Input: part model. Units: mm. Frame: model coordinates. A direction names the side the tool comes from. Coordinates: 2 decimals unless noted, no trailing zeros. Loops run counter-clockwise (first coordinate to the right, second up) from the corner with the lowest first, then second, coordinate; pieces in that order, holes last. Notation, with made-up numbers: (48, -10.5) -> (107, -10.5) arc R22 ccw to (107, 26.5) -> close; hole circle Ø7 at (-32.75, 14.5). An arc over 180 degrees is marked (long way). Answer as a JSON object with one key per item and string values.
from build123d import *

# Parameters (mm, degrees)
BOSS_EXTRUDE1_DEPTH  = 1
SKETCH2_W            = 16
SKETCH2_H            = 10
BOSS_EXTRUDE2_DEPTH  = 10
SKETCH3_W            = 4.889113018
SKETCH3_H            = 5.37802432
CUT_EXTRUDE1_DEPTH   = 10
SKETCH4_W            = 45
SKETCH4_H            = 2.4
SKETCH4_W_2          = 30
BOSS_EXTRUDE3_DEPTH  = 4
SKETCH5_W            = 35
SKETCH5_H            = 10
BOSS_EXTRUDE4_DEPTH  = 7
SKETCH6_W            = 35
SKETCH6_H            = 1.5
CUT_EXTRUDE2_DEPTH   = 4
FILLET1_R            = 1
SKETCH7_R            = 1.5
CUT_EXTRUDE3_DEPTH   = 4
SKETCH8_W            = 0.75
SKETCH8_H            = 0.75
BOSS_EXTRUDE5_DEPTH  = 6
LPATTERN1_COUNT      = 10
LPATTERN1_PITCH      = 3
SKETCH9_W            = 0.75
SKETCH9_H            = 0.75
BOSS_EXTRUDE6_DEPTH  = 6
LPATTERN2_COUNT      = 15
LPATTERN2_PITCH      = 3
SKETCH10_R           = 2.5
BOSS_EXTRUDE7_DEPTH  = 6
SKETCH11_W           = 4.8
SKETCH11_H           = 9
BOSS_EXTRUDE8_DEPTH  = 4
SKETCH12_W           = 0.75
SKETCH12_H           = 0.75
BOSS_EXTRUDE9_DEPTH  = 6
LPATTERN3_COUNT      = 3
LPATTERN3_PITCH      = 3
LPATTERN3_COUNT_DIR2 = 2
LPATTERN3_PITCH_DIR2 = 3
SKETCH13_W           = 14.120912951
SKETCH13_H           = 4.362558473
BOSS_EXTRUDE10_DEPTH = 4
FILLET2_R            = 1


with BuildPart() as part:
    # Sketch1 → Boss-Extrude1 (new body)
    with BuildSketch(Plane.XY):
        Polygon((22.754016647, 124.270947632), (19.754016647, 127.270947632), (-45.245983353, 127.270947632), (-45.245983353, 74.270947632), (19.754016647, 74.270947632), (19.754016647, 90.113910289), (22.754016647, 92.500164177), align=None)
    extrude(amount=-BOSS_EXTRUDE1_DEPTH)

    # Sketch2 → Boss-Extrude2 (add)
    with BuildSketch(Plane(origin=(0, 0, -1), x_dir=(-1, 0, 0), z_dir=(0, 0, -1))):
        with Locations((46.316496684, 91.208096568)):
            Rectangle(SKETCH2_W, SKETCH2_H)
    extrude(amount=BOSS_EXTRUDE2_DEPTH)

    # Sketch3 → Cut-Extrude1 (cut)
    with BuildSketch(Plane.ZY.offset(54.316496684)):
        with Locations((-6.06540843, 91.2419286)):
            Rectangle(SKETCH3_W, SKETCH3_H)
    extrude(amount=-CUT_EXTRUDE1_DEPTH, mode=Mode.SUBTRACT)

    # Sketch4 → Boss-Extrude3 (add)
    with BuildSketch(Plane(origin=(0, 0, -1), x_dir=(-1, 0, 0), z_dir=(0, 0, -1))):
        with Locations((5.745983353, 77.470947632)):
            Rectangle(SKETCH4_W, SKETCH4_H)
        with Locations((-0.254016647, 124.070947632)):
            Rectangle(SKETCH4_W_2, SKETCH4_H)
    extrude(amount=BOSS_EXTRUDE3_DEPTH)

    # Sketch5 → Boss-Extrude4 (add)
    with BuildSketch(Plane(origin=(0, 0, -1), x_dir=(-1, 0, 0), z_dir=(0, 0, -1))):
        with Locations((3.745983353, 113.370947632)):
            Rectangle(SKETCH5_W, SKETCH5_H)
    extrude(amount=BOSS_EXTRUDE4_DEPTH)

    # Sketch6 → Cut-Extrude2 (cut)
    with BuildSketch(Plane(origin=(0, 0, -8), x_dir=(-1, 0, 0), z_dir=(0, 0, -1))):
        with Locations((3.745983353, 117.620947632)):
            Rectangle(SKETCH6_W, SKETCH6_H)
        with Locations((3.745983353, 109.120947632)):
            Rectangle(SKETCH6_W, SKETCH6_H)
    extrude(amount=-CUT_EXTRUDE2_DEPTH, mode=Mode.SUBTRACT)

    # Fillet1
    fillet1_edges = [part.edges().sort_by_distance(p)[0] for p in [
        (13.754016647, 109.870947632, -6),
        (-21.245983353, 109.870947632, -6),
        (13.754016647, 116.870947632, -6),
        (-21.245983353, 116.870947632, -6),
    ]]
    fillet(fillet1_edges, radius=FILLET1_R)

    # Sketch7 → Cut-Extrude3 (cut)
    with BuildSketch(Plane(origin=(0, 0, -1), x_dir=(-1, 0, 0), z_dir=(0, 0, -1))):
        with Locations((-17.700101194, 119.270947632)):
            Circle(SKETCH7_R)
        with Locations((-17.700101194, 91.270947632)):
            Circle(SKETCH7_R)
        with Locations((33.799898806, 125.270947632)):
            Circle(SKETCH7_R)
        with Locations((33.799898806, 77.270947632)):
            Circle(SKETCH7_R)
    extrude(amount=-CUT_EXTRUDE3_DEPTH, mode=Mode.SUBTRACT)

    # Sketch8 → Boss-Extrude5 (add)
    with BuildSketch(Plane(origin=(0, 0, -5), x_dir=(-1, 0, 0), z_dir=(0, 0, -1))):
        with Locations((-13.879016647, 124.070947632)):
            Rectangle(SKETCH8_W, SKETCH8_H)
    boss_extrude5 = extrude(amount=BOSS_EXTRUDE5_DEPTH)

    # LPattern1: Boss-Extrude5 ×10
    with Locations(*[(-i * LPATTERN1_PITCH, 0, 0) for i in range(1, LPATTERN1_COUNT)]):
        add(boss_extrude5)

    # Sketch9 → Boss-Extrude6 (add)
    with BuildSketch(Plane(origin=(0, 0, -5), x_dir=(-1, 0, 0), z_dir=(0, 0, -1))):
        with Locations((-15.402792453, 77.470947632)):
            Rectangle(SKETCH9_W, SKETCH9_H)
    boss_extrude6 = extrude(amount=BOSS_EXTRUDE6_DEPTH)

    # LPattern2: Boss-Extrude6 ×15
    with Locations(*[(-i * LPATTERN2_PITCH, 0, 0) for i in range(1, LPATTERN2_COUNT)]):
        add(boss_extrude6)

    # Sketch10 → Boss-Extrude7 (add)
    with BuildSketch(Plane(origin=(0, 0, -1), x_dir=(-1, 0, 0), z_dir=(0, 0, -1))):
        with Locations((26.546732083, 118.214976991)):
            Circle(SKETCH10_R)
        with Locations((31.940661119, 118.214976991)):
            Circle(SKETCH10_R)
    extrude(amount=BOSS_EXTRUDE7_DEPTH)

    # Sketch11 → Boss-Extrude8 (add)
    with BuildSketch(Plane(origin=(0, 0, -1), x_dir=(-1, 0, 0), z_dir=(0, 0, -1))):
        with Locations((-19.349242758, 100.613910289)):
            Rectangle(SKETCH11_W, SKETCH11_H)
    extrude(amount=BOSS_EXTRUDE8_DEPTH)

    # Sketch12 → Boss-Extrude9 (add)
    with BuildSketch(Plane(origin=(0, 0, -5), x_dir=(-1, 0, 0), z_dir=(0, 0, -1))):
        with Locations((-20.624242758, 97.488910289)):
            Rectangle(SKETCH12_W, SKETCH12_H)
    boss_extrude9 = extrude(amount=BOSS_EXTRUDE9_DEPTH)

    # LPattern3: Boss-Extrude9 3 × 2
    with Locations(*[(-j * LPATTERN3_PITCH_DIR2, i * LPATTERN3_PITCH, 0) for i in range(LPATTERN3_COUNT) for j in range(LPATTERN3_COUNT_DIR2) if (i, j) != (0, 0)]):
        add(boss_extrude9)

    # Sketch13 → Boss-Extrude10 (add)
    with BuildSketch(Plane(origin=(0, 0, -1), x_dir=(-1, 0, 0), z_dir=(0, 0, -1))):
        with Locations((23.447660741, 101.747194556)):
            Rectangle(SKETCH13_W, SKETCH13_H)
    extrude(amount=BOSS_EXTRUDE10_DEPTH)

    # Fillet2
    fillet2_edges = [part.edges().sort_by_distance(p)[0] for p in [
        (-16.387204265, 103.928473792, -3),
        (-16.387204265, 99.565915319, -3),
        (-30.508117216, 99.565915319, -3),
        (-30.508117216, 103.928473792, -3),
    ]]
    fillet(fillet2_edges, radius=FILLET2_R)


solid = part.part
1. Section query C-C (y = 95). Return loops of the section in (x, z).
Reply:
{"outline": "(-54.32, -11) -> (-38.32, -11) -> (-38.32, -1) -> (22.75, -1) -> (22.75, 0) -> (-45.25, 0) -> (-45.25, -1) -> (-54.32, -1) -> close"}
2. Section query A-A (x = -40). Return loops of the section in (y, z), plus the area to 3 significant figures.
Reply:
{"outline": "(74.27, -1) -> (86.21, -1) -> (86.21, -11) -> (96.21, -11) -> (96.21, -1) -> (127.27, -1) -> (127.27, 0) -> (74.27, 0) -> close", "area": "153 mm2"}
3. Line query: line 1 along Y through (x, z) = (2.5, -2); line 2 along X through (y, z) = (117, -3); line 3 along X through (y, z) = (100.5, -6.5). Output: solid intervals per line, ascending.
Reply:
{"line 1": "y = 76.27 to 78.67, 108.37 to 118.37, 122.87 to 125.27", "line 2": "x = -34.13 to -29.76, -28.73 to -24.36, -21.25 to 13.75", "line 3": "x = 17.25 to 18, 20.25 to 21"}
4. Section query D-D (y = 122). Return loops of the section in (x, z).
Reply:
{"outline": "(-45.25, -1) -> (22.75, -1) -> (22.75, 0) -> (-45.25, 0) -> close"}
5. Section query B-B (z = -9.5). Count the separate pieces of the cut face and the enclosed holes in it, plus the area to 3 significant figures.
Reply:
{"separate pieces": "32", "enclosed holes": "0", "area": "177 mm2"}
6. Access query for faces 4 (the face through (16.949, 101, -3)), 5 (the face through (-49, 91, -8.51)), 6 (the face through (-26.005, 115.774, -3.958)). Directions: +Z, -Z, +X, -X, +Y, -Y. A direction counts if a zero-diameter tool reaches every point of the face in a straight line with its end or side. Return the directions, or none.
Reply:
{"face 4": "-Z, +Y, -Y", "face 5": "-X", "face 6": "-Z"}
7. Pin query (flat end, axial travel): P1, Ø0.8, axis at x = 5, z = -8.5, coming from the -Y side; P2, Ø10, axis at x = 12.5, y = 85, coming from the +Z side; P3, Ø0.6, axis at x = -14.5, z = -7.5, coming from the -Y side; P4, Ø6, axis at x = -34, y = 89.5, coming from the -Z side. Return the tip coordinate at first contact, or that it passes through.
Reply:
{"P1": "stops at y = 123.7", "P2": "stops at z = 0", "P3": "stops at y = 77.1", "P4": "stops at z = -1"}
8. Mould query, pull axis Y, two halves, no side actions, for faces 1 (the face through (-30.508, 102, -3)), 2 (the face through (21.23, 91.29, -0.49)), 3 (the face through (-5, 78.671, -3)). Classes: pulls with the +Y half, pulls with the -Y half, needs draft (parallel to the pull), parting line crosses it, or undercut.
Reply:
{"face 1": "needs draft", "face 2": "pulls with the -Y half", "face 3": "undercut"}
